```python
from build123d import *

# Parameters (mm, degrees)
TROU_TARAUD_M31_D            = 2.5
R_P_TITION_CIRCULAIRE1_COUNT = 4
CHANFREIN1_SIZE              = 0.2
CONG_1_R                     = 2


with BuildPart() as part:
    # Esquisse1 → Révolution1 (revolve)
    with BuildSketch(Plane(origin=(0, 0, 0), x_dir=(0, 0, -1), z_dir=(1, 0, 0))):
        Polygon((-9, -2), (-9, 0), (-10.5, 0), (-10.5, 5), (-17.5, 5), (-17.5, -2), align=None)
    revolve(axis=Axis((0, 0, 0), (0, -1, 0)))

    # Trou taraudé M31 (through all)
    with Locations(Plane(origin=(0, 5, 0), x_dir=(-1, 0, 0), z_dir=(0, 1, 0))):
        with Locations((0, -14)):
            trou_taraud_m31 = Hole(TROU_TARAUD_M31_D / 2)

    # Répétition circulaire1: Trou taraudé M31 ×4 about axis
    r_p_tition_circulaire1_axis = Axis((0, 0, 0), (0, 1, 0))
    for i in range(1, R_P_TITION_CIRCULAIRE1_COUNT):
        add(trou_taraud_m31.rotate(r_p_tition_circulaire1_axis, i * 360 / R_P_TITION_CIRCULAIRE1_COUNT), mode=Mode.SUBTRACT)

    # Chanfrein1
    chanfrein1_edges = [part.edges().sort_by_distance(p)[0] for p in [
        (0, 5, -17.5),
        (0, 5, -10.5),
    ]]
    chamfer(chanfrein1_edges, length=CHANFREIN1_SIZE)

    # Congé1
    cong_1_edges = [part.edges().sort_by_distance(p)[0] for p in [
        (0, -2, -17.5),
    ]]
    fillet(cong_1_edges, radius=CONG_1_R)


solid = part.part
```
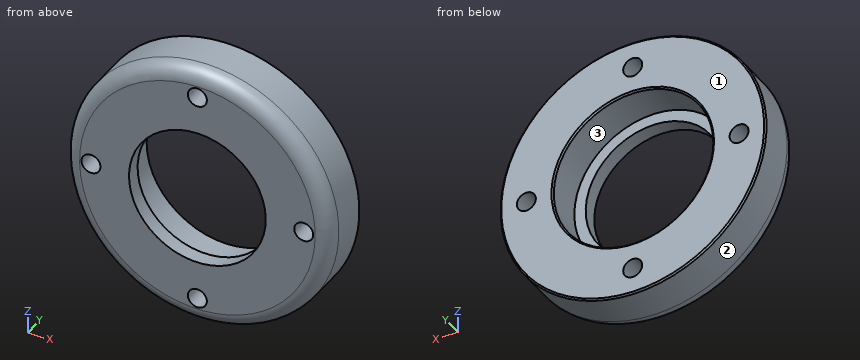
The model under review builds one solid part; all positions refer to its coordinate system, in mm. Face numbers are marked on the shaded views. Round coordinates to 2 decimals unless told otherwise and drop trailing zeros. Order: outer loops, then holes, each group sorted by start corner. A loop starts at its lowest first (then second) coordinate and runs counter-clockwise, first axis right, second up. Notation, with made-up numbers: (-20.75, 85.5) -> (-16.75, 85.5) arc R17 cw to (-16.75, 106.5) -> close; hole circle Ø8 at (17.5, 74.5). An arc over 180 degrees is marked (long way). One line per item, written item: value. Start each with the question number.
Q1. Clearance check with flat-ended pins moving along their axes: pin 1 Ø20.5 at (x, z) = (0, 0) entering from +Y; pin 2 Ø2 at (y, z) = (-1, 5) entering from -X; pin 3 Ø4 at (x, y) = (11, 2.5) entering from +Z; pin 4 Ø6.5 at (x, z) = (3.5, -1.5) entering from +Y. State where each tip first meets the part, or that it passes through.
Q2. Mouldability with a two-part tool opening along X and no side actions: class the marked faces 1, 2 and 3 as released by +X, released by -X, zero draft, split by the parting line, or undercut.
Q3. Take a section at B-B (y = 4). Write out the cut boundary in (x, z).
Q4. Take a section at A-A (x = 0). Write out the cut boundary in (y, z).
Q5. Wall thickness on line 1 (Z direction, x = 0, y = 2.75); line 2 (Z direction, x = 9, y = 4.5): over which ranges is each line inside the solid? List them lowest first.
Q6. Take a section at C-C (y = -1.5). Write out the cut boundary in (x, z).
Reported:
1. pin 1: stops at y = 0
1. pin 2: stops at x = -16.95
1. pin 3: stops at z = 15.01
1. pin 4: passes through
2. face 1: zero draft
2. face 2: split by the parting line
2. face 3: undercut
3. outline: circle Ø35 at (0, 0); hole circle Ø2.5 at (-14, 0); hole circle Ø21 at (0, 0); hole circle Ø2.5 at (0, -14); hole circle Ø2.5 at (0, 14); hole circle Ø2.5 at (14, 0)
4. outline: (-2, -15.5) arc R2 ccw to (0, -17.5) -> (4.8, -17.5) -> (5, -17.3) -> (5, -15.25) -> (-2, -15.25) -> close; (-2, -12.75) -> (5, -12.75) -> (5, -10.7) -> (4.8, -10.5) -> (0, -10.5) -> (0, -9) -> (-2, -9) -> close; (-2, 9) -> (0, 9) -> (0, 10.5) -> (4.8, 10.5) -> (5, 10.7) -> (5, 12.75) -> (-2, 12.75) -> close; (-2, 15.25) -> (5, 15.25) -> (5, 17.3) -> (4.8, 17.5) -> (0, 17.5) arc R2 ccw to (-2, 15.5) -> close
5. line 1: z = -17.5 to -15.25, -12.75 to -10.5, 10.5 to 12.75, 15.25 to 17.5
5. line 2: z = -15.01 to -5.41, 5.41 to 15.01
6. outline: circle Ø33.65 at (0, 0); hole circle Ø2.5 at (-14, 0); hole circle Ø18 at (0, 0); hole circle Ø2.5 at (0, -14); hole circle Ø2.5 at (0, 14); hole circle Ø2.5 at (14, 0)
